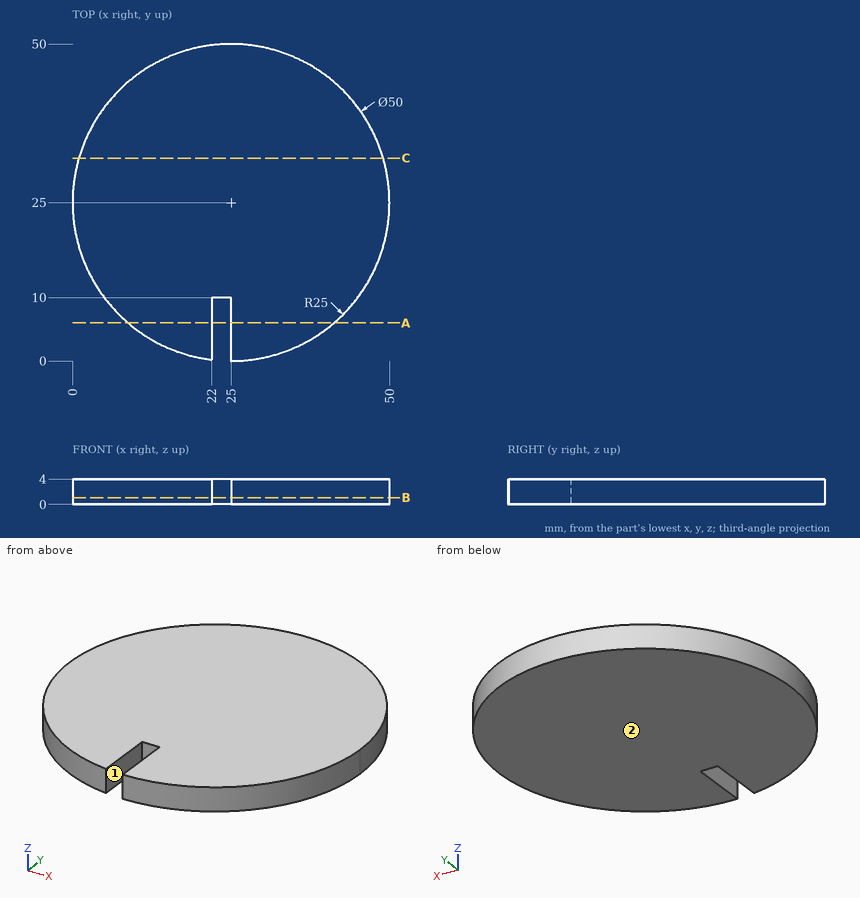
Design review of the part shown in the three views and the two pictorial views. Dimensions are in mm from the part's minimum x, y and z. Give positions to 0.01 mm unless a question says otherwise; leave off trailing zeros. Write each loop counter-clockwise with the first axis right and the second up, starting at its lowest first coordinate (ties: lowest second). Pieces come first, ordered by that corner, then holes. Notation, with made-up numbers: (19, 52) -> (25, 52) arc R10 ccw to (25, 62) -> close; hole circle Ø3 at (82, 24.25). An arc over 180 degrees is marked (long way). Answer in a Markdown table with one row per item.
1) Add section C-C on y = 32. State the section outline as (x, z) points, plus the area to 3 significant figures.
Worked answers:
| item | result |
|---|---|
| outline | (1, 0) -> (49, 0) -> (49, 4) -> (1, 4) -> close |
| area | 192 mm² |
2) For L1, parallel to X at y = 16, z = 3.7; L2, parallel to X at y = 40, z = 1.95; L3, parallel to Y at x = 37, z = 3.4, list the stretches that pass through material, from the lowest coordinate up. Write a range as [from, to].
Worked answers:
| item | result |
|---|---|
| L1 | [1.68, 48.32] |
| L2 | [5, 45] |
| L3 | [3.07, 46.93] |
3) Add section B-B on z = 1.05. State the section outline as (x, y) points, plus the area to 3 significant figures.
Worked answers:
| item | result |
|---|---|
| outline | (22, 0.18) -> (22, 10) -> (25, 10) -> (25, 0) arc R25 ccw (long way) to start |
| area | 1,930 mm² |
4) Clearance check with flat-ended pins moving along their axes: P1, Ø1.5, axis at y = 19.5, z = 3.5, coming from the -X side; P2, Ø1.2, axis at y = 5, z = 1, coming from the -X side. State where each tip first meets the part, or that it passes through.
Worked answers:
| item | result |
|---|---|
| P1 | x = 0.46 |
| P2 | x = 9.23 |
5) Add section A-A on y = 6. State the section outline as (x, z) points.
Worked answers:
| item | result |
|---|---|
| outline | (8.75, 0) -> (22, 0) -> (22, 4) -> (8.75, 4) -> close; (25, 0) -> (41.25, 0) -> (41.25, 4) -> (25, 4) -> close |
6) Mouldability with a two-part tool opening along X and no side actions: class the marked faces 1 and 2 as +X half, -X half, draft (parallel to the pull), parting line (faces both ways), or undercut.
Worked answers:
| item | result |
|---|---|
| face 1 | undercut |
| face 2 | draft |
